The figure shows three views and two pictorial views of one solid part (mm, origin at its lowest corner). Answer the questions. Round coordinates to 2 decimals unless told otherwise and drop trailing zeros. Write each loop counter-clockwise with the first axis right and the second up, starting at its lowest first coordinate (ties: lowest second). Pieces come first, ordered by that corner, then holes. Notation, with made-up numbers: M 85.25,37.25 L 109.25,37.25 A15 cw 109.25,46.25 Z; hole C 40,6.5 d3. An arc over 180 degrees is marked long. Answer in a Markdown table with one row per item.
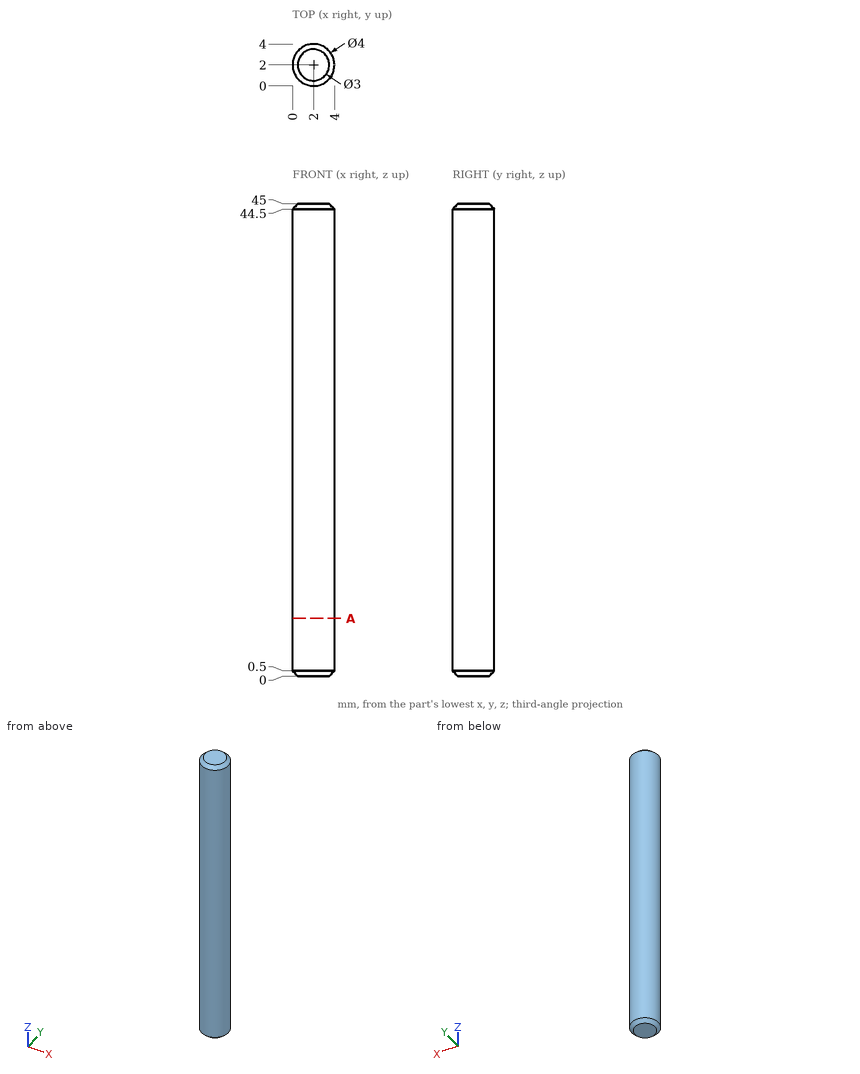
1. The part is cut by section A-A (z = 5.5). Determine the outline of the cut face in (x, y).
Calculated:
| item | result |
|---|---|
| outline | C 2,2 d4 |
2. Consider line 1 along X through (y, z) = (3.75, 15); line 2 along X through (y, z) = (1.25, 41); line 3 along Y through (x, z) = (1.4, 29.5). Determine where each line is inside the solid, lowest interval first. Write a range as from..to.
Calculated:
| item | result |
|---|---|
| line 1 | x = 1.03..2.97 |
| line 2 | x = 0.15..3.85 |
| line 3 | y = 0.09..3.91 |
3. Given pin 1 (1 mm diameter, centred on x = 0.5, z = 6.5, fed in from +Y), flat-ended and moving along its own axis, determine where the tip first touches the part or whether it passes through.
Calculated:
| item | result |
|---|---|
| pin 1 | stops at y = 3.73 |
